CAD build for the part. Positions are in the model's coordinates, mm. Face numbers are marked on the shaded views. A direction names the side the tool comes from. Round coordinates to 2 decimals unless told otherwise and drop trailing zeros. Order: outer loops, then holes, each group sorted by start corner. A loop starts at its lowest first (then second) coordinate and runs counter-clockwise, first axis right, second up.
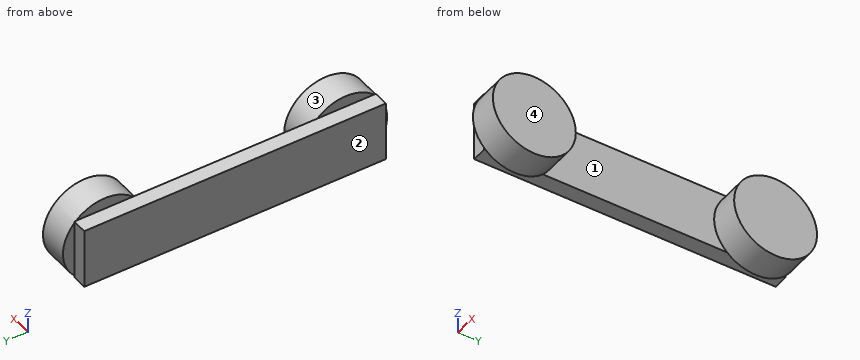
```python
from build123d import *

# Parameters (mm, degrees)
SKETCH1_W           = 50.8
SKETCH1_H           = 254
BOSS_EXTRUDE1_DEPTH = 6.35
SKETCH2_R           = 34.925
BOSS_EXTRUDE2_DEPTH = 25.4


with BuildPart() as part:
    # Sketch1 → Boss-Extrude1 (new, symmetric)
    with BuildSketch(Plane(origin=(0, 0, 0), x_dir=(0, 0, -1), z_dir=(1, 0, 0))):
        Rectangle(SKETCH1_W, SKETCH1_H)
    extrude(amount=BOSS_EXTRUDE1_DEPTH, both=True)

    # Sketch2 → Boss-Extrude2 (add)
    with BuildSketch(Plane(origin=(6.35, 0, 0), x_dir=(0, 0, -1), z_dir=(1, 0, 0))):
        with Locations(Location((0, 101.6, 0), (0, 0, 223.341758227))):
            Circle(SKETCH2_R)
        with Locations(Location((0, -101.6, 0), (0, 0, 136.658241773))):
            Circle(SKETCH2_R)
    extrude(amount=BOSS_EXTRUDE2_DEPTH)


solid = part.part
```
1. Mould opens along Y. For the marked faces 1 and 2 say: released by +Y, released by -Y, zero draft, split by the parting line, or undercut.
2. Cut at D-D, the plane z = -28.5. Write the cut outline in (x, y), and give its area (3 significant figures).
3. Drill centre lines: line 1 (Z direction, x = -1.5, y = -16.5); line 2 (X direction, y = -12, z = -13.5); line 3 (Y direction, x = 13.5, z = -8). Where is each one in solid material? Low to high.
4. Cut at C-C, the plane z = 0. Write the cut outline in (x, y) (3 decimals).
5. Cut at B-B, the plane x = 9. Write the cut outline in (y, z) (3 decimals), and give its area (3 significant figures).
6. Pin check, flat tips, straight feed: P1, Ø1, axis at x = 27.5, z = 13, coming from the +Y side; P2, Ø6.5, axis at x = -0.5, y = -63.5, coming from the -Z side; P3, Ø1.5, axis at x = 26, z = 18.5, coming from the -Y side; P4, Ø4, axis at x = 10, y = -22.5, coming from the -Z side. Stop position of each tip, or through.
7. Tool access for the marked faces 3 and 4: list every direction of +Z, -Z, +X, -X, +Y, -Y with a clear straight run to the whole face (end or side of a thin tool).
8. Cut at A-A, the plane y = -101.6. Write the cut outline in (x, z) (3 decimals), and give its area (3 significant figures).
Outcome:
1. face 1: undercut
1. face 2: zero draft
2. outline: (6.35, -121.79) - (31.75, -121.79) - (31.75, -81.41) - (6.35, -81.41) - close; (6.35, 81.41) - (31.75, 81.41) - (31.75, 121.79) - (6.35, 121.79) - close
2. area: 2,050 mm2
3. line 1: z = -25.4 to 25.4
3. line 2: x = -6.35 to 6.35
3. line 3: y = -135.6 to -67.6, 67.6 to 135.6
4. outline: (-6.35, -127) - (6.35, -127) - (6.35, -136.525) - (31.75, -136.525) - (31.75, -66.675) - (6.35, -66.675) - (6.35, 66.675) - (31.75, 66.675) - (31.75, 136.525) - (6.35, 136.525) - (6.35, 127) - (-6.35, 127) - close
5. outline: circle Ø69.85 at (-101.6, 0); circle Ø69.85 at (101.6, 0)
5. area: 7,660 mm2
6. P1: stops at y = 134.21
6. P2: stops at z = -25.4
6. P3: stops at y = -131.68
6. P4: passes through
7. face 3: +X
7. face 4: +Z, -Z, +X, +Y, -Y
8. outline: (-6.35, -25.4) - (6.35, -25.4) - (6.35, -34.925) - (31.75, -34.925) - (31.75, 34.925) - (6.35, 34.925) - (6.35, 25.4) - (-6.35, 25.4) - close
8. area: 2,420 mm2
